from build123d import *

# Parameters (mm, degrees)
ESQUISSE1_R             = 40
BOSS_EXTRU_1_DEPTH      = 4
ESQUISSE2_R             = 38
BOSS_EXTRU_2_DEPTH      = 8
BOSS_EXTRU_2_DEPTH_BACK = 12
CHANFREIN1_SIZE         = 1
ESQUISSE3_R             = 2.1
ENL_V_MAT_EXTRU_1_DEPTH = 21


with BuildPart() as part:
    # Esquisse1 → Boss.-Extru.1 (new body)
    with BuildSketch(Plane.XY):
        Circle(ESQUISSE1_R)
    extrude(amount=BOSS_EXTRU_1_DEPTH)

    # Esquisse2 → Boss.-Extru.2 (add, two sides)
    with BuildSketch(Plane.XY.offset(4)) as boss_extru_2_sk:
        Circle(ESQUISSE2_R)
    extrude(amount=BOSS_EXTRU_2_DEPTH)
    extrude(boss_extru_2_sk.sketch, amount=-BOSS_EXTRU_2_DEPTH_BACK)

    # Chanfrein1
    chanfrein1_edges = [part.edges().sort_by_distance(p)[0] for p in [
        (-38, 0, -8),
        (-38, 0, 12),
    ]]
    chamfer(chanfrein1_edges, length=CHANFREIN1_SIZE)

    # Esquisse3 → Enlèv. mat.-Extru.1 (cut, through all)
    with BuildSketch(Plane.XY.offset(12)):
        with Locations((25, 0)):
            Circle(ESQUISSE3_R)
        with Locations((-25, 0)):
            Circle(ESQUISSE3_R)
    extrude(amount=-ENL_V_MAT_EXTRU_1_DEPTH, mode=Mode.SUBTRACT)


solid = part.part
Here's how the part is built. I have some questions about the finished solid (model axes, mm). A direction names the side the tool comes from. Round coordinates to 2 decimals unless told otherwise and drop trailing zeros. Loops run counter-clockwise (first coordinate to the right, second up) from the corner with the lowest first, then second, coordinate; pieces in that order, holes last. Notation, with made-up numbers: M -15.75,7.25 L 19.25,7.25 A37 cw 19.25,46.25 Z; hole C -25,74 d3. An arc over 180 degrees is marked long. Write each question's results on one line, items separated by ' | '. Start each with the question number.
(1) I want a section at C-C (x = 0). Please give me the cut outline in (y, z).
(2) Thinking about a two-plate mould opening in X: for faces 4 (the flat face through (-1, 1, -8)), 5 (the cylindrical face through (27.003, 0.631, 2.14)), 6 (the cylindrical face through (-8.67, -39.05, 1.97)), which applies, pulls with the +X half, pulls with the -X half, needs draft (parallel to the pull), parting line crosses it, or undercut?
(3) On a 3-axis mill with a long thin cutter (end or side, diameter ignored), from which of +Z, -Z, +X, -X, +Y, -Y can I reach the whole of each face in a straight line? I mean faces 1 (the cylindrical face through (17.535, -33.713, 7.451)), 2 (the cylindrical face through (-22.997, 0.631, 2.14)), 3 (the flat face through (35.4, -14.6, 0)). Say none if no direction works.
(4) I want a section at A-A (y = 0). Please give me the cut outline in (x, z).
(5) Will these pins go through, and if not, where does the flat tip stop? P1, Ø4, axis at x = 11.5, z = -0.5, coming from the -Y side; P2, Ø1.5, axis at y = -8.5, z = 6, coming from the +X side; P3, Ø2.5, axis at x = 25, y = 0, coming from the -Z side; P4, Ø8, axis at x = -7, z = 0.5, coming from the +Y side.
(6) I want a section at B-B (z = -2.75). Please give me the cut outline in (x, y), then the cut area to 3 significant figures.
(7) If I drill on probe 1 along Y at (x, z) = (24, 5.5); probe 2 along Y at (x, z) = (25, -1.75); probe 3 along X at (y, z) = (-12.5, 3), over which ranges is the centre line in solid material (lowest first)? Write a range as from..to.
Solved:
1) outline: M -40,0 L -38,0 L -38,-7 L -37,-8 L 37,-8 L 38,-7 L 38,0 L 40,0 L 40,4 L 38,4 L 38,11 L 37,12 L -37,12 L -38,11 L -38,4 L -40,4 Z
2) face 4: needs draft | face 5: undercut | face 6: parting line crosses it
3) face 1: +Z | face 2: +Z, -Z | face 3: -Z
4) outline: M -40,0 L -38,0 L -38,-7 L -37,-8 L -27.1,-8 L -27.1,12 L -37,12 L -38,11 L -38,4 L -40,4 Z; M -22.9,-8 L 22.9,-8 L 22.9,12 L -22.9,12 Z; M 27.1,-8 L 37,-8 L 38,-7 L 38,0 L 40,0 L 40,4 L 38,4 L 38,11 L 37,12 L 27.1,12 Z
5) P1: stops at y = -38.84 | P2: stops at x = 37.2 | P3: passes through | P4: stops at y = 39.89
6) outline: C 0,0 d76; hole C -25,0 d4.2; hole C 25,0 d4.2 | area: 4,510 mm²
7) probe 1: y = -29.46..-1.85, 1.85..29.46 | probe 2: y = -28.62..-2.1, 2.1..28.62 | probe 3: x = -38..38
